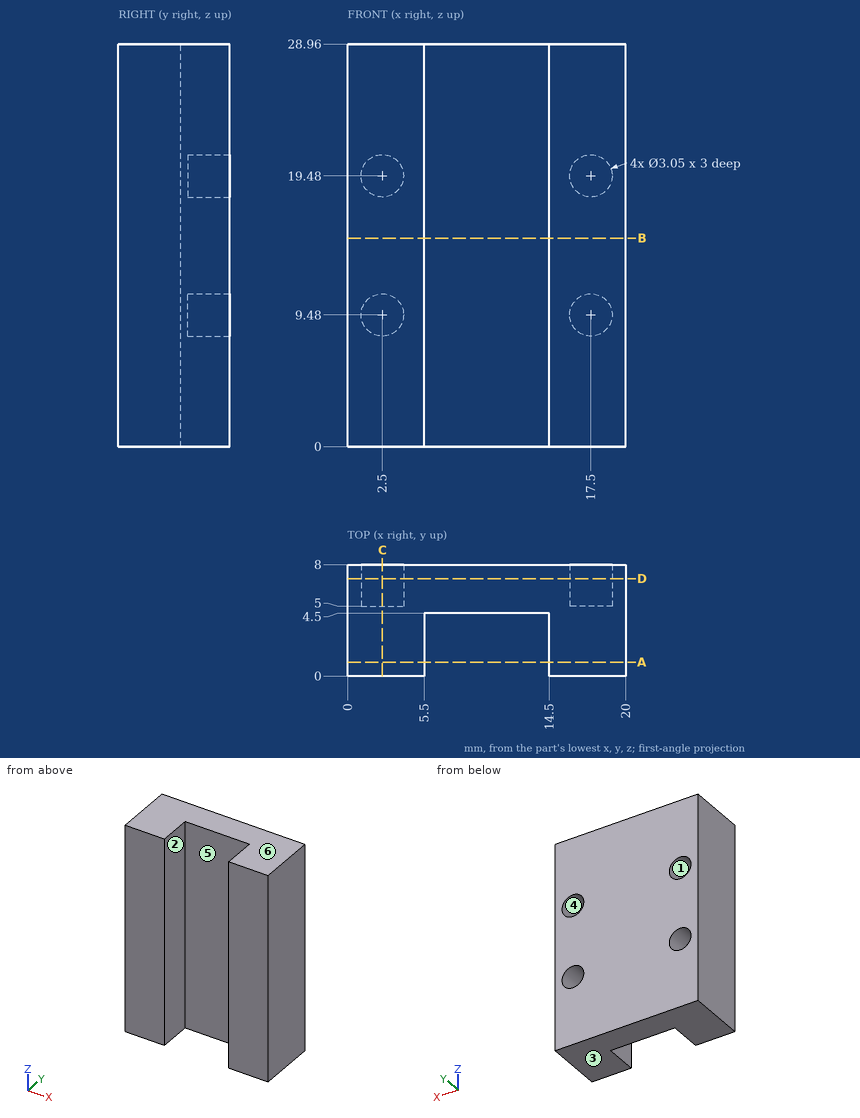
Could you check a few things on this drawing? It's one solid part, dimensions in mm from its lowest x, y, z. A direction names the side the tool comes from. Round coordinates to 2 decimals unless told otherwise and drop trailing zeros. Write each loop counter-clockwise with the first axis right and the second up, starting at its lowest first coordinate (ties: lowest second). Pieces come first, ordered by that corner, then holes. Notation, with made-up numbers: (13.25, 16.25) -> (19.25, 16.25) arc R14 cw to (19.25, 41.25) -> close; hole circle Ø7 at (-31.5, 27.5). An arc over 180 degrees is marked (long way). Use a Markdown table: item, result.
1. We'd pull the mould along Z, two halves only. Please class the marked faces 1, 2 and 3: +Z half, -Z half, draft (parallel to the pull), parting line (faces both ways), or undercut.
Answer key:
| item | result |
|---|---|
| face 1 | undercut |
| face 2 | draft |
| face 3 | -Z half |
2. If we section it at D-D (y = 7): List the corners of the cut face in (x, z) for me (3 decimals), then the cut area to 3 significant figures.
Answer key:
| item | result |
|---|---|
| outline | (0, 0) -> (20, 0) -> (20, 28.96) -> (0, 28.96) -> close; hole circle Ø3.05 at (2.5, 9.48); hole circle Ø3.05 at (2.5, 19.48); hole circle Ø3.05 at (17.5, 9.48); hole circle Ø3.05 at (17.5, 19.48) |
| area | 550 mm^2 |
3. If we section it at B-B (z = 15): List the corners of the cut face in (x, y) for me.
Answer key:
| item | result |
|---|---|
| outline | (0, 0) -> (5.5, 0) -> (5.5, 4.5) -> (14.5, 4.5) -> (14.5, 0) -> (20, 0) -> (20, 8) -> (0, 8) -> close |
4. Please list where these lines run through material, in increasing order: probe 1 along Z at (x, y) = (17.5, 7) (3 decimals); probe 2 along X at (y, z) = (2, 18); probe 3 along Z at (x, y) = (17, 7).
Answer key:
| item | result |
|---|---|
| probe 1 | z = 0 to 7.955, 11.005 to 17.955, 21.005 to 28.96 |
| probe 2 | x = 0 to 5.5, 14.5 to 20 |
| probe 3 | z = 0 to 8.04, 10.92 to 18.04, 20.92 to 28.96 |
5. For pin 1 Ø1.5 at (x, z) = (2.5, 19.5) entering from +Y; pin 2 Ø1.5 at (x, y) = (8, 1) entering from -Z, each with a flat end and sliding along its axis, tell me the tip position at first contact or that it passes through.
Answer key:
| item | result |
|---|---|
| pin 1 | stops at y = 5 |
| pin 2 | passes through |
6. If we section it at C-C (x = 2.5): List the corners of the cut face in (y, z) for me (3 decimals), then the cut area to 3 significant figures.
Answer key:
| item | result |
|---|---|
| outline | (0, 0) -> (8, 0) -> (8, 7.955) -> (5, 7.955) -> (5, 11.005) -> (8, 11.005) -> (8, 17.955) -> (5, 17.955) -> (5, 21.005) -> (8, 21.005) -> (8, 28.96) -> (0, 28.96) -> close |
| area | 213 mm^2 |
7. If we section it at A-A (y = 1): List the corners of the cut face in (x, z) for me, then the cut area to 3 significant figures.
Answer key:
| item | result |
|---|---|
| outline | (0, 0) -> (5.5, 0) -> (5.5, 28.96) -> (0, 28.96) -> close; (14.5, 0) -> (20, 0) -> (20, 28.96) -> (14.5, 28.96) -> close |
| area | 319 mm^2 |
8. Which directions (+Z, -Z, +X, -X, +Y, -Y) give clear straight access to the entire face, cutting with the end or side of a thin tool? Please do the marked faces 4, 5 and 6.
Answer key:
| item | result |
|---|---|
| face 4 | +Y |
| face 5 | +Z, -Z, -Y |
| face 6 | +Z, +X, -X, +Y, -Y |
